Geometry check sheet. Reference: the model listing, model coordinates, mm. A direction names the side the tool comes from. Coordinates: 2 decimals unless noted, no trailing zeros. Loops run counter-clockwise (first coordinate to the right, second up) from the corner with the lowest first, then second, coordinate; pieces in that order, holes last. Notation, with made-up numbers: (62.25, -10.75) -> (115.25, -10.75) arc R25 ccw to (115.25, 4.25) -> close; hole circle Ø11 at (25, 86). An arc over 180 degrees is marked (long way). Answer as a JSON object with one key per item and string values.
from build123d import *

# Parameters (mm, degrees)
ESQUISSE1_R                = 2.75
BOSS_EXTRU_1_DEPTH         = 3
ESQUISSE2_W                = 15
ESQUISSE2_H                = 25
BOSS_EXTRU_2_DEPTH         = 6
R_P_TITION_LIN_AIRE1_COUNT = 3
R_P_TITION_LIN_AIRE1_PITCH = 6.5
BOSS_EXTRU_3_DEPTH         = 3
ENL_V_MAT_EXTRU_1_DEPTH    = 3
ESQUISSE4_3_R              = 1.75
ENL_V_MAT_EXTRU_3_DEPTH    = 31.809901006


with BuildPart() as part:
    # Esquisse1 → Boss.-Extru.1 (new body)
    with BuildSketch(Plane.XY):
        with BuildLine():
            Line((0, 0), (15, 0))
            Line((15, 0), (15, 8))
            ThreePointArc((15, 8), (7.5, 15.5), (0, 8))
            Line((0, 8), (0, 0))
        make_face()
        with Locations((7.5, 8)):
            Circle(ESQUISSE1_R, mode=Mode.SUBTRACT)
    boss_extru_1 = extrude(amount=BOSS_EXTRU_1_DEPTH)

    # Esquisse2 → Boss.-Extru.2 (add)
    with BuildSketch(Plane.XZ):
        with Locations((7.5, -9.5)):
            Rectangle(ESQUISSE2_W, ESQUISSE2_H)
    boss_extru_2 = extrude(amount=BOSS_EXTRU_2_DEPTH)

    # R_p_tition lin_aire1: Boss.-Extru.1 ×3
    with Locations(*[(0, 0, -i * R_P_TITION_LIN_AIRE1_PITCH) for i in range(1, R_P_TITION_LIN_AIRE1_COUNT)]):
        add(boss_extru_1)

    # Esquisse3 → Boss.-Extru.3 (add)
    with BuildSketch(Plane.XY.offset(3)):
        with BuildLine():
            Line((0, 8), (0, -6))
            Line((0, -6), (15, -6))
            Line((15, -6), (15, 8))
            ThreePointArc((15, 8), (7.5, 15.5), (0, 8))
        make_face()
        Polygon((9.780533563, 4.05), (12.061067127, 8), (9.780533563, 11.95), (5.219466437, 11.95), (2.938932873, 8), (5.219466437, 4.05), align=None, mode=Mode.SUBTRACT)
    extrude(amount=BOSS_EXTRU_3_DEPTH)

    # Esquisse4 → Enl_v. mat.-Extru.1 (cut)
    with BuildSketch(Plane(origin=(0, 0, 0), x_dir=(1, 0, 0), z_dir=(0, 1, 0))):
        Polygon((9.116580754, 14.7), (10.733161507, 17.5), (9.116580754, 20.3), (5.883419246, 20.3), (4.266838493, 17.5), (5.883419246, 14.7), align=None)
    enl_v_mat_extru_1 = extrude(amount=-ENL_V_MAT_EXTRU_1_DEPTH, mode=Mode.SUBTRACT)

    # Esquisse4_3 → Enl_v. mat.-Extru.3 (cut, through all)
    with BuildSketch(Plane(origin=(0, 0, 0), x_dir=(1, 0, 0), z_dir=(0, 1, 0))):
        with Locations(Location((7.5, 17.5, 0), (0, 0, 270))):
            Circle(ESQUISSE4_3_R)
    enl_v_mat_extru_3 = extrude(amount=-ENL_V_MAT_EXTRU_3_DEPTH, mode=Mode.SUBTRACT)

    # Sym_trie1: Boss.-Extru.2, Enl_v. mat.-Extru.1, Enl_v. mat.-Extru.3 across plane
    add(boss_extru_2.mirror(Plane(origin=(0, 0, -3.5), x_dir=(1, 0, 0), z_dir=(0, 0, -1))))
    add(enl_v_mat_extru_1.mirror(Plane(origin=(0, 0, -3.5), x_dir=(1, 0, 0), z_dir=(0, 0, -1))), mode=Mode.SUBTRACT)
    add(enl_v_mat_extru_3.mirror(Plane(origin=(0, 0, -3.5), x_dir=(1, 0, 0), z_dir=(0, 0, -1))), mode=Mode.SUBTRACT)


solid = part.part
1. Section check B-B, the plane y = 10.25. Record the boundary of the cut face in (x, z).
Evaluation:
{"outline": "(0.35, -13) -> (5.92, -13) -> (5.92, -10) -> (0.35, -10) -> close; (0.35, -6.5) -> (5.92, -6.5) -> (5.92, -3.5) -> (0.35, -3.5) -> close; (0.35, 0) -> (5.92, 0) -> (5.92, 3) -> (4.24, 3) -> (4.24, 6) -> (0.35, 6) -> close; (9.08, -13) -> (14.65, -13) -> (14.65, -10) -> (9.08, -10) -> close; (9.08, -6.5) -> (14.65, -6.5) -> (14.65, -3.5) -> (9.08, -3.5) -> close; (9.08, 0) -> (14.65, 0) -> (14.65, 6) -> (10.76, 6) -> (10.76, 3) -> (9.08, 3) -> close"}
2. Depth check by flat-ended pin: P1, Ø7.5, axis at x = 9.5, y = 11.5, coming from the -Z side; P2, Ø4.5, axis at x = 6.5, z = 10, coming from the +Y side; P3, Ø6.5, axis at x = 7.5, y = 8, coming from the +Z side. Enter the tip coordinate at first touch or a pass-through.
Evaluation:
{"P1": "stops at z = -13", "P2": "stops at y = 0", "P3": "stops at z = 3"}
3. Section check C-C, the plane x = 7.5. State how many separate pieces and enclosed holes the cut face has, then the cut area to 3 significant figures.
Evaluation:
{"separate pieces": "6", "enclosed holes": "0", "area": "280 mm^2"}
4. Thickness scan on probe 1 along Z at (x, y) = (3, 5.25); probe 2 along Z at (x, y) = (4.5, 9.75); probe 3 along Y at (x, z) = (7.5, -4.45). Record the ranges inside material, lowest first. Write a range as from..to.
Evaluation:
{"probe 1": "z = -13..-10, -6.5..-3.5, 0..6", "probe 2": "z = -13..-10, -6.5..-3.5, 0..3", "probe 3": "y = -6..5.25, 10.75..15.5"}
5. Mould release check, pull along X, two halves, no side actions. Record for faces 4 (the face through (0, -0.5, -3.2)), 5 (the face through (7, -3, 15)), 6 (the face through (7, -1, 7.7)): released by +X, released by -X, zero draft, split by the parting line, or undercut.
Evaluation:
{"face 4": "released by -X", "face 5": "zero draft", "face 6": "undercut"}
6. Section check D-D, the plane z = -8. Record the boundary of the cut face in (x, y).
Evaluation:
{"outline": "(0, -6) -> (15, -6) -> (15, 0) -> (0, 0) -> close"}
7. Section check A-A, the plane y = 3. Record the boundary of the cut face in (x, z).
Evaluation:
{"outline": "(0, -13) -> (15, -13) -> (15, -10) -> (0, -10) -> close; (0, -6.5) -> (15, -6.5) -> (15, -3.5) -> (0, -3.5) -> close; (0, 0) -> (15, 0) -> (15, 6) -> (0, 6) -> close"}
8. Tool access check on faces 1 (the face through (11, 4, 6)), 2 (the face through (4.095, 10.003, 4.479)), 3 (the face through (9, -3, -19)). Record the directions out of +Z, -Z, +X, -X, +Y, -Y that give a thin tool (end or side, any length) a straight path to the whole face; none if there is none.
Evaluation:
{"face 1": "+Z, +X, -X, +Y", "face 2": "+Z", "face 3": "+Y"}
